```python
from build123d import *

# Parameters (mm, degrees)
SKETCH2_R             = 22.5
SKETCH2_R_2           = 16.9
BOSS_EXTRUDE1_DEPTH   = 19
SKETCH2_R_3           = 36
SKETCH2_R_4           = 27
BOSS_EXTRUDE1_2_DEPTH = 19
BOSS_EXTRUDE2_DEPTH   = 9
CUT_EXTRUDE1_DEPTH    = 4
CUT_EXTRUDE2_DEPTH    = 99
BOSS_EXTRUDE3_DEPTH   = 30
CUT_EXTRUDE3_START    = -99
SKETCH6_R             = 27
CUT_EXTRUDE3_DEPTH    = 99
SKETCH7_R             = 4.5
CUT_EXTRUDE4_DEPTH    = 99


with BuildPart() as part:
    # Sketch2 → Boss-Extrude1 (new, symmetric)
    with BuildSketch(Plane.XY):
        Circle(SKETCH2_R)
        Circle(SKETCH2_R_2, mode=Mode.SUBTRACT)
    extrude(amount=BOSS_EXTRUDE1_DEPTH, both=True)



with BuildPart() as body_2:
    # Sketch2 → Boss-Extrude1 2 (new, symmetric)
    with BuildSketch(Plane.XY):
        with Locations((0, -201.2)):
            Circle(SKETCH2_R_3)
        with Locations((0, -201.2)):
            Circle(SKETCH2_R_4, mode=Mode.SUBTRACT)
    extrude(amount=BOSS_EXTRUDE1_2_DEPTH, both=True)


with BuildPart() as part_1:
    add(part.part)

    add(body_2.part)  # Boss-Extrude2 merges body 2
    # Sketch2<5> → Boss-Extrude2 (add, symmetric)
    with BuildSketch(Plane.XY):
        with BuildLine():
            Line((0, -165.2), (0, -22.5))
            ThreePointArc((0, -22.5), (-5.135562367, -21.906072199), (-10, -20.155644371))
            Line((-10, -20.155644371), (-23.469590176, -173.902045187))
            ThreePointArc((-23.469590176, -173.902045187), (-12.515462971, -167.445545677), (0, -165.2))
        make_face()
        with BuildLine():
            ThreePointArc((10, -20.155644371), (5.135562367, -21.906072199), (0, -22.5))
            Line((0, -22.5), (0, -165.2))
            ThreePointArc((0, -165.2), (12.515462971, -167.445545677), (23.469590176, -173.902045187))
            Line((23.469590176, -173.902045187), (10, -20.155644371))
        make_face()
    extrude(amount=BOSS_EXTRUDE2_DEPTH, both=True)

    # Sketch3 → Cut-Extrude1 (cut)
    with BuildSketch(Plane.XY.offset(9)):
        with BuildLine():
            Line((8, -55.6), (8, -145.6))
            ThreePointArc((8, -145.6), (0, -153.6), (-8, -145.6))
            Line((-8, -145.6), (-8, -55.6))
            ThreePointArc((-8, -55.6), (0, -47.6), (8, -55.6))
        make_face()
    cut_extrude1 = extrude(amount=-CUT_EXTRUDE1_DEPTH, mode=Mode.SUBTRACT)

    # Mirror1: Cut-Extrude1 across plane
    add(cut_extrude1.mirror(Plane.XY), mode=Mode.SUBTRACT)

    # Sketch4 → Cut-Extrude2 (cut)
    with BuildSketch(Plane.XY.offset(19)):
        Polygon((0, -201.2), (-54.705364776, -201.2), (-51.550648926, -248.976612299), (37.861738866, -255.19137468), (50.544643276, -201.2), align=None)
    extrude(amount=-CUT_EXTRUDE2_DEPTH, mode=Mode.SUBTRACT)

    # Sketch5 → Boss-Extrude3 (add)
    with BuildSketch(Plane(origin=(0, -171.2, 0), x_dir=(-1, 0, 0), z_dir=(0, -1, 0))):
        with BuildLine():
            Line((38, -9), (-38, -9))
            ThreePointArc((-38, -9), (-47, 0), (-38, 9))
            Line((-38, 9), (38, 9))
            ThreePointArc((38, 9), (47, 0), (38, -9))
        make_face()
    extrude(amount=BOSS_EXTRUDE3_DEPTH)

    # Sketch6 → Cut-Extrude3 (cut)
    with BuildSketch(Plane.XY.offset(9).offset(CUT_EXTRUDE3_START)):
        with Locations((0, -201.2)):
            Circle(SKETCH6_R)
    extrude(amount=CUT_EXTRUDE3_DEPTH, mode=Mode.SUBTRACT)

    # Sketch7 → Cut-Extrude4 (cut)
    with BuildSketch(Plane(origin=(0, -171.2, 0), x_dir=(1, 0, 0), z_dir=(0, 1, 0))):
        with Locations(Location((38, 0, 0), (0, 0, 270))):
            Circle(SKETCH7_R)
    cut_extrude4 = extrude(amount=-CUT_EXTRUDE4_DEPTH, mode=Mode.SUBTRACT)

    # Mirror2: Cut-Extrude4 across plane
    add(cut_extrude4.mirror(Plane(origin=(0, 0, 0), x_dir=(0, 0, 1), z_dir=(1, 0, 0))), mode=Mode.SUBTRACT)


solid = part_1.part
```
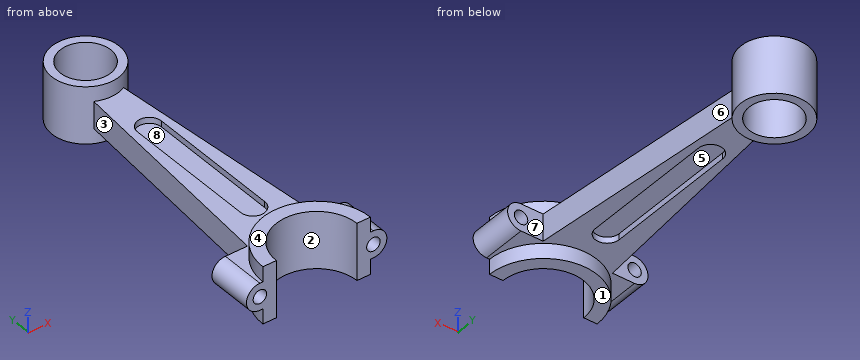
Here's how the part is built. I have some questions about the finished solid (model axes, mm). Face numbers are marked on the shaded views. A direction names the side the tool comes from. Give positions to 0.01 mm unless a question says otherwise; leave off trailing zeros. Order: outer loops, then holes, each group sorted by start corner. A loop starts at its lowest first (then second) coordinate and runs counter-clockwise, first axis right, second up. Notation, with made-up numbers: M 74.5,74.25 L 90.5,74.25 A20 ccw 90.5,96.25 Z; hole C 1.25,-7.75 d1. An arc over 180 degrees is marked long. Use a Markdown table: item, result. Add a question column.
1. On a 3-axis mill with a long thin cutter (end or side, diameter ignored), from which of +Z, -Z, +X, -X, +Y, -Y can I reach the whole of each face in a straight line? I mean the marked faces 4, 5, 6, 7 and 8. Say none if no direction works.
2. Suppose I cut it at D-D (y = -90.5). List the corners of the cut face in (x, z) for me, and give its area (3 significant figures).
3. For pin 1 Ø5 at (x, y) = (15, -111.5) entering from -Z; pin 2 Ø3 at (y, z) = (-84, -8) entering from +X; pin 3 Ø5 at (x, y) = (3, -120) entering from -Z; pin 4 Ø10.5 at (x, z) = (38, 0) entering from -Y, each with a flat end and sliding along its axis, tell me the tip position at first contact or that it passes through.
4. Suppose I cut it at B-B (z = 13). List the corners of the cut face in (x, y) for me, and give its area (3 significant figures).
5. I need wall thicknesses on probe 1 along X at (y, z) = (-191, 0); probe 2 along X at (y, z) = (-184.25, 0); probe 3 along Z at (x, y) = (-38, -185). Which ranges of each line are inside material? Lowest first, please. Write a range as from..to.
6. If we mould it in two halves opening along Y, with no side actions, what happens to the marked faces 1, 2 and 3? For each: +Y half, -Y half, draft (parallel to the pull), parting line (faces both ways), or undercut.
7. Suppose I cut it at A-A (z = 0). List the corners of the cut face in (x, y) for me.
8. Suppose I cut it at C-C (x = 6). List the corners of the cut face in (y, z) for me.
Results list:
| question | item | result |
|---|---|---|
| 1 | face 4 | +Z, +X, -X, +Y, -Y |
| 1 | face 5 | -Z |
| 1 | face 6 | +Z, -Z, +X |
| 1 | face 7 | +Z, -Z, +X, +Y |
| 1 | face 8 | +Z |
| 2 | outline | M -16.16,-9 L -8,-9 L -8,-5 L 8,-5 L 8,-9 L 16.16,-9 L 16.16,9 L 8,9 L 8,5 L -8,5 L -8,9 L -16.16,9 Z |
| 2 | area | 454 mm² |
| 3 | pin 1 | stops at z = -9 |
| 3 | pin 2 | stops at x = 15.72 |
| 3 | pin 3 | stops at z = -5 |
| 3 | pin 4 | stops at y = -201.2 |
| 4 | outline | M -36,-201.2 L -27,-201.2 A27 cw 27,-201.2 L 36,-201.2 A36 ccw Z; C 0,0 d45; hole C 0,0 d33.8 |
| 4 | area | 1,580 mm² |
| 5 | probe 1 | x = -47..-42.5, -33.5..-25, 25..33.5, 42.5..47 |
| 5 | probe 2 | x = -47..-42.5, -33.5..-21.02, 21.02..33.5, 42.5..47 |
| 5 | probe 3 | z = -9..-4.5, 4.5..9 |
| 6 | face 1 | draft |
| 6 | face 2 | -Y half |
| 6 | face 3 | undercut |
| 7 | outline | M -47,-201.2 L -42.5,-201.2 L -42.5,-171.2 L -47,-171.2 Z; M -33.5,-201.2 L -27,-201.2 A27 cw 27,-201.2 L 33.5,-201.2 L 33.5,-171.2 L 23.23,-171.2 L 10,-20.16 A22.5 ccw long -10,-20.16 L -23.23,-171.2 L -33.5,-171.2 Z; M 42.5,-201.2 L 47,-201.2 L 47,-171.2 L 42.5,-171.2 Z; hole C 0,0 d33.8 |
| 8 | outline | M -174.88,-19 L -165.7,-19 L -165.7,-9 L -150.89,-9 L -150.89,-5 L -50.31,-5 L -50.31,-9 L -21.69,-9 L -21.69,-19 L -15.8,-19 L -15.8,19 L -21.69,19 L -21.69,9 L -50.31,9 L -50.31,5 L -150.89,5 L -150.89,9 L -165.7,9 L -165.7,19 L -174.88,19 Z; M 15.8,-19 L 21.69,-19 L 21.69,19 L 15.8,19 Z |
